```python
from build123d import *

# Parameters (mm, degrees)
F0_W     = 38.1
F0_H     = 88.9
F1_DEPTH = 609.6
F2_R     = 6.35
F3_DEPTH = 38.1
F4_R     = 76.2
F5_R     = 5.08


with BuildPart() as f1:
    # F0 (on Front) → F1 (new body)
    with BuildSketch(Plane.XZ):
        Rectangle(F0_W, F0_H)
    extrude(amount=-F1_DEPTH)

    # F2 (on face) → F3 (cut)
    with BuildSketch(Plane(origin=(-19.05, 0, 0), x_dir=(0, -1, 0), z_dir=(-1, 0, 0))):
        with Locations((-410.6418, 14.732)):
            Circle(F2_R)
        with Locations((-410.6418, -14.732)):
            Circle(F2_R)
        with Locations((-364.1598, 14.732)):
            Circle(F2_R)
        with Locations((-364.1598, -14.732)):
            Circle(F2_R)
    extrude(amount=-F3_DEPTH, mode=Mode.SUBTRACT)

    # F4
    f4_edges = [f1.edges().sort_by_distance(p)[0] for p in [
        (0, 609.6, 44.45),
        (0, 0, 44.45),
    ]]
    fillet(f4_edges, radius=F4_R)

    # F5
    f5_edges = [f1.edges().sort_by_distance(p)[0] for p in [
        (-19.05, 304.8, 44.45),
        (19.05, 304.8, 44.45),
    ]]
    fillet(f5_edges, radius=F5_R)


solid = f1.part
```
Could you check a few things on this model? Use its own coordinates, in mm. Coordinates: 2 decimals unless noted, no trailing zeros. Order: outer loops, then holes, each group sorted by start corner. A loop starts at its lowest first (then second) coordinate and runs counter-clockwise, first axis right, second up. Notation, with made-up numbers: M -7,78 L 37,78 A15 ccw 37,96 Z; hole C 55.25,-30 d8. An arc over 180 degrees is marked long. Use a Markdown table: item, result. Add a question column.
Q1. We'd pull the mould along Z, two halves only. Please class faces 1 (the flat face through (19.05, 301, -3)), 2 (the cylindrical face through (0.196, 587.871, 21.536)), 3 (the cylindrical face through (-0.267, 404.776, 12.3)): pulls with the +Z half, pulls with the -Z half, needs draft (parallel to the pull), parting line crosses it, or undercut.
Q2. I want a section at A-A on x = 3. List the corners of the cut face in (y, z) for me.
Q3. If I drill on L1, parallel to Z at x = 7, y = 364.5; L2, parallel to Y at x = 2, z = -20; L3, parallel to Y at x = 0.5, z = 9.5, over which ranges is the centre line in solid material (lowest first)?
Q4. I'm going to push flat-ended pins straight in: pin 1 (3 mm diameter, centred on x = -8, z = 13.5, fed in from -Y); pin 2 (12 mm diameter, centred on x = 5, z = -2, fed in from -Y); pin 3 (1.5 mm diameter, centred on x = -13.5, z = -26.5, fed in from +Y). Where does each tip first touch, or does it pass through?
Checked values:
| question | item | result |
|---|---|---|
| 1 | face 1 | needs draft |
| 1 | face 2 | pulls with the +Z half |
| 1 | face 3 | undercut |
| 2 | outline | M 0,-44.45 L 609.6,-44.45 L 609.6,-31.75 A76.2 ccw 533.4,44.45 L 76.2,44.45 A76.2 ccw 0,-31.75 Z; hole C 364.16,-14.73 d12.7; hole C 364.16,14.73 d12.7; hole C 410.64,-14.73 d12.7; hole C 410.64,14.73 d12.7 |
| 3 | L1 | -44.45 to -21.07, -8.39 to 8.39, 21.07 to 44.45 |
| 3 | L2 | 0.91 to 360.61, 367.71 to 407.1, 414.19 to 608.69 |
| 3 | L3 | 12.13 to 360.56, 367.76 to 407.04, 414.24 to 597.47 |
| 4 | pin 1 | y = 13.81 |
| 4 | pin 2 | y = 3.8 |
| 4 | pin 3 | y = 609.47 |
